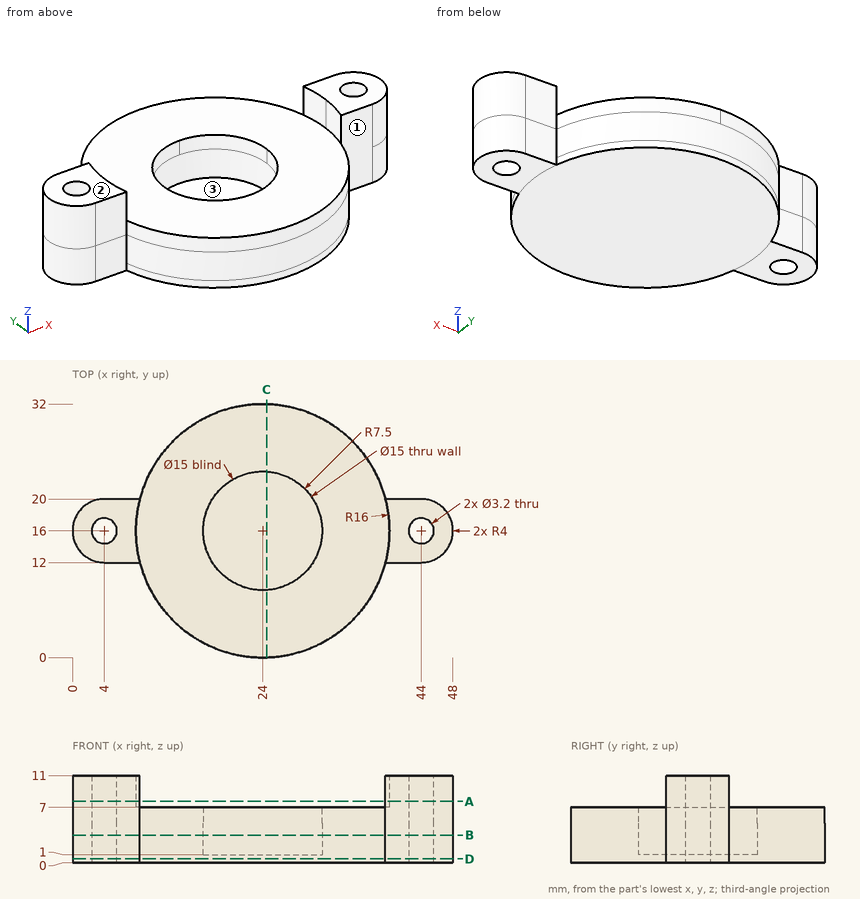
Part print with two shaded views. Sizes in mm from the minimum x, y, z corner. A direction names the side the tool comes from. Coordinates: 2 decimals unless noted, no trailing zeros. Write each loop counter-clockwise with the first axis right and the second up, starting at its lowest first coordinate (ties: lowest second). Pieces come first, ordered by that corner, then holes.
1. 3-axis set-ups, long thin cutter, end or side, ignore diameter. For the marked faces 1, 2 and 3: which of +Z, -Z, +X, -X, +Y, -Y reach the whole face in a straight line?
Answer block:
face 1: +Z, -Z, +X, -Y
face 2: +Z, +X, -X, +Y, -Y
face 3: +Z
2. Band-saw the part on D-D, the plane z = 0.5. Give the cut face in (x, y), and give its area (3 significant figures).
Answer block:
outline: (4, 12) - (8.51, 12) arc R16 ccw to (39.49, 12) - (44, 12) arc R4 ccw to (44, 20) - (39.49, 20) arc R16 ccw to (8.51, 20) - (4, 20) arc R4 ccw to start; hole circle Ø3.2 at (4, 16); hole circle Ø3.2 at (44, 16)
area: 905 mm2
3. Band-saw the part on B-B, the plane z = 3.5. Give the cut face in (x, y), and give its area (3 significant figures).
Answer block:
outline: (4, 12) - (8.51, 12) arc R16 ccw to (39.49, 12) - (44, 12) arc R4 ccw to (44, 20) - (39.49, 20) arc R16 ccw to (8.51, 20) - (4, 20) arc R4 ccw to start; hole circle Ø3.2 at (4, 16); hole circle Ø15 at (24, 16); hole circle Ø3.2 at (44, 16)
area: 728 mm2
4. Band-saw the part on A-A, the plane z = 7.75. Give the cut face in (x, y), and give its area (3 significant figures).
Answer block:
outline: (4, 12) - (8.51, 12) arc R16 cw to (8.51, 20) - (4, 20) arc R4 ccw to start; (39.49, 12) - (44, 12) arc R4 ccw to (44, 20) - (39.49, 20) arc R16 cw to start; hole circle Ø3.2 at (4, 16); hole circle Ø3.2 at (44, 16)
area: 101 mm2
5. Band-saw the part on C-C, the plane x = 24.5. Give the cut face in (y, z), and give its area (3 significant figures).
Answer block:
outline: (0.01, 0) - (31.99, 0) - (31.99, 7) - (23.48, 7) - (23.48, 1) - (8.52, 1) - (8.52, 7) - (0.01, 7) - close
area: 134 mm2
6. Drop flat-ended pins along their axis: pin 1 (3 mm diameter, centred on y = 9.5, z = 9, fed in from +X); pin 2 (16.5 mm diameter, centred on x = 25.5, y = 13, fed in from +Z); pin 3 (2.5 mm diameter, centred on x = 6, z = 3.5, fed in from +Y); pin 4 (3.5 mm diameter, centred on x = 5, z = 8.5, fed in from -Y). Give the stop position or say it passes through.
Answer block:
pin 1: passes through
pin 2: stops at z = 7
pin 3: stops at y = 20
pin 4: stops at y = 12
7. Drill centre lines: probe 1 along Y at (x, z) = (44, 2.8); probe 2 along X at (y, z) = (16.5, 1.5); probe 3 along Y at (x, z) = (24, 4.2). Where is each one in solid material? Low to high.
Answer block:
probe 1: y = 12 to 14.4, 17.6 to 20
probe 2: x = 0.03 to 2.48, 5.52 to 16.52, 31.48 to 42.48, 45.52 to 47.97
probe 3: y = 0 to 8.5, 23.5 to 32
